Part model, mm, in its own coordinate system. A direction names the side the tool comes from. Coordinates: 2 decimals unless noted, no trailing zeros. Write each loop counter-clockwise with the first axis right and the second up, starting at its lowest first coordinate (ties: lowest second). Pieces come first, ordered by that corner, then holes. Notation, with made-up numbers: M 37,2 L 42,2 A35 ccw 42,37 Z; hole C 62.5,48.5 d9. An arc over 180 degrees is marked long. Use a Markdown table: item, result. Add a question column.
Q1. Slice it at D-D on y = -21.5. Write the cut outline in (x, z), then the cut area to 3 significant figures.
Q2. Tool access for faces 4 (the cylindrical face through (16.631, -22.476, 5.014)), 5 (the flat face through (-9, -34, 6)): list every direction of +Z, -Z, +X, -X, +Y, -Y with a clear straight run to the whole face (end or side of a thin tool).
Q3. Wall check: L1, parallel to X at y = -71.5, z = 4.5; L2, parallel to Y at x = 0, z = 1; L3, parallel to Y at x = 7, z = 5. Give the ranges that are in metal, low to high. Write a range as from..to.
Q4. Slice it at B-B on x = 0. Write the cut outline in (y, z).
Q5. Slice it at C-C on z = 2.25. Write the cut outline in (x, y).
Q6. Pin check, flat tip, straight feed: pin 1 Ø1.8 at (x, y) = (16.85, -21.5) entering from +Z. Stop position of the tip, or through.
Q7. Mould opens along Y. For faces 1 (the cylindrical face through (17.309, -72.387, 5.014)), 2 (the flat face through (0, -85, 3)), 3 (the flat face through (-20, -36, 3)) say: released by +Y, released by -Y, zero draft, split by the parting line, or undercut.
Q8. Slice it at A-A on y = 0. Write the cut outline in (x, z), then the cut area to 3 significant figures.
from build123d import *

# Parameters (mm, degrees)
F0_W     = 40
F0_H     = 100
F0_R     = 11
F1_DEPTH = 6
F3_START = 16.5
F2_R     = 12.25
F3_DEPTH = 60
F4_R     = 1
F5_DEPTH = 2


with BuildPart() as f1:
    # F0 (on Top) → F1 (new body)
    with BuildSketch(Plane.XY):
        with Locations((0, -35)):
            Rectangle(F0_W, F0_H)
        Circle(F0_R, mode=Mode.SUBTRACT)
    extrude(amount=F1_DEPTH)

    # F2 (on Front) → F3 (cut)
    with BuildSketch(Plane.XZ.offset(F3_START)):
        with Locations((0, 17.25)):
            Circle(F2_R)
    extrude(amount=F3_DEPTH, mode=Mode.SUBTRACT)

    # F4 (on face) → F5 (cut)
    with BuildSketch(Plane.XY.offset(6)):
        with Locations((-16.8476798574, -21.5)):
            Circle(F4_R)
        with Locations((16.8476798574, -21.5)):
            Circle(F4_R)
        with Locations((-16.8476798574, -71.5)):
            Circle(F4_R)
        with Locations((16.8476798574, -71.5)):
            Circle(F4_R)
    extrude(amount=-F5_DEPTH, mode=Mode.SUBTRACT)


solid = f1.part
Recorded:
| question | item | result |
|---|---|---|
| 1 | outline | M -20,0 L 20,0 L 20,6 L 17.85,6 L 17.85,4 L 15.85,4 L 15.85,6 L 4.85,6 A12.25 cw -4.85,6 L -15.85,6 L -15.85,4 L -17.85,4 L -17.85,6 L -20,6 Z |
| 1 | area | 225 mm² |
| 2 | face 4 | +Z |
| 2 | face 5 | +Z, +X, -X, +Y, -Y |
| 3 | L1 | -20..-17.85, -15.85..15.85, 17.85..20 |
| 3 | L2 | -85..-11, 11..15 |
| 3 | L3 | -85..-8.49, 8.49..15 |
| 4 | outline | M -85,0 L -11,0 L -11,6 L -16.5,6 L -16.5,5 L -76.5,5 L -76.5,6 L -85,6 Z; M 11,0 L 15,0 L 15,6 L 11,6 Z |
| 5 | outline | M -20,-85 L 20,-85 L 20,15 L -20,15 Z; hole C 0,0 d22 |
| 6 | pin 1 | z = 4 |
| 7 | face 1 | undercut |
| 7 | face 2 | released by -Y |
| 7 | face 3 | zero draft |
| 8 | outline | M -20,0 L -11,0 L -11,6 L -20,6 Z; M 11,0 L 20,0 L 20,6 L 11,6 Z |
| 8 | area | 108 mm² |
